Build history of the part. All positions in model axes, mm. A direction names the side the tool comes from. Give positions to 0.01 mm unless a question says otherwise; leave off trailing zeros. Loops run counter-clockwise (first coordinate to the right, second up) from the corner with the lowest first, then second, coordinate; pieces in that order, holes last. Notation, with made-up numbers: (14, 81) -> (30, 81) arc R33 cw to (30, 115) -> close; hole circle Ø6 at (-10, 44). An arc over 180 degrees is marked (long way). Answer as a JSON object with one key per item and string values. Group by question number.
Q1. Two-plate mould, pull along Y, no slides. Class faces 1 (the cylindrical face through (-77.91, 51.38, 25.76)), 2 (the flat face through (-4, 3, 0)), 3 (the flat face through (-76.156, 3, 27)): pulls with the +Y half, pulls with the -Y half, needs draft (parallel to the pull), parting line crosses it, or undercut.
Q2. Band-saw the part on B-B, the plane y = 8. Write the cut outline in (x, z) (3 decimals), plus the area to 3 significant figures.
Q3. Wall check: probe 1 along X at (y, z) = (-44, 37.5); probe 2 along Y at (x, z) = (-60, 47.5); probe 3 along X at (y, z) = (42, 43). Give the ranges that are in metal, low to high. Write a range as from..to.
Q4. Drop flat-ended pins along their axis: pin 1 (2 mm diameter, centred on x = 7.5, y = -9, fed in from +Z) (3 decimals); pin 2 (3 mm diameter, centred on x = -57, y = 26.5, fed in from -Z). Give the stop position or say it passes through.
Q5. Band-saw the part on C-C, the plane x = 63. Write the cut outline in (y, z) (3 decimals), plus the area to 3 significant figures.
Q6. Band-saw the part on A-A, the plane z = 40. Write the cut outline in (x, y) (3 decimals), plus the area to 3 significant figures.
Q7. Tool access for faces 4 (the flat face through (73.069, 1, 25)), 5 (the flat face through (-2, 49.712, 27)): list every direction of +Z, -Z, +X, -X, +Y, -Y with a clear straight run to the whole face (end or side of a thin tool).
from build123d import *

# Parameters (mm, degrees)
F1_DEPTH = 50.8
F2_R     = 5
F3_T     = -3.175


with BuildPart() as f1:
    # F0 (on Top) → F1 (new body)
    with BuildSketch(Plane.XY):
        Polygon((73.068974, -48.712649), (-79.331026, 52.887351), (-79.331026, -48.712649), align=None)
        Polygon((73.068974, 52.887351), (-79.331026, 52.887351), (73.068974, -48.712649), align=None)
    extrude(amount=F1_DEPTH)

    # F2
    f2_edges = [f1.edges().sort_by_distance(p)[0] for p in [
        (-79.331026, -48.712649, 25.4),
        (73.068974, -48.712649, 25.4),
        (73.068974, 52.887351, 25.4),
        (-79.331026, 52.887351, 25.4),
    ]]
    fillet(f2_edges, radius=F2_R)

    # F3
    f3_openings = [f1.faces().sort_by_distance(p)[0] for p in [
        (-3.131026, 2.087351, 50.8),
    ]]
    offset(amount=F3_T, openings=f3_openings)


solid = f1.part
Worked answers:
{
 "1": {"face 1": "pulls with the +Y half", "face 2": "needs draft", "face 3": "undercut"},
 "2": {"outline": "(-79.331, 0) -> (73.069, 0) -> (73.069, 50.8) -> (69.894, 50.8) -> (69.894, 3.175) -> (-76.156, 3.175) -> (-76.156, 50.8) -> (-79.331, 50.8) -> close", "area": "786 mm2"},
 "3": {"probe 1": "-79.32..-76.13, 69.87..73.06", "probe 2": "-48.71..-45.54, 49.71..52.89", "probe 3": "-79.33..-76.16, 69.89..73.07"},
 "4": {"pin 1": "z = 3.175", "pin 2": "z = 0"},
 "5": {"outline": "(-48.713, 0) -> (52.887, 0) -> (52.887, 50.8) -> (49.712, 50.8) -> (49.712, 3.175) -> (-45.538, 3.175) -> (-45.538, 50.8) -> (-48.713, 50.8) -> close", "area": "625 mm2"},
 "6": {"outline": "(-79.331, -43.713) arc R5 ccw to (-74.331, -48.713) -> (68.069, -48.713) arc R5 ccw to (73.069, -43.713) -> (73.069, 47.887) arc R5 ccw to (68.069, 52.887) -> (-74.331, 52.887) arc R5 ccw to (-79.331, 47.887) -> close; hole (-76.156, -43.713) arc R1.825 ccw to (-74.331, -45.538) -> (68.069, -45.538) arc R1.825 ccw to (69.894, -43.713) -> (69.894, 47.887) arc R1.825 ccw to (68.069, 49.712) -> (-74.331, 49.712) arc R1.825 ccw to (-76.156, 47.887) -> close", "area": "1,550 mm2"},
 "7": {"face 4": "+Z, -Z, +X, +Y, -Y", "face 5": "+Z"}
}
